Build history of the part. All positions in model axes, mm. A direction names the side the tool comes from. Round coordinates to 2 decimals unless told otherwise and drop trailing zeros. Write each loop counter-clockwise with the first axis right and the second up, starting at its lowest first coordinate (ties: lowest second). Pieces come first, ordered by that corner, then holes. Notation, with made-up numbers: (-5, 84) -> (1, 84) arc R5 cw to (1, 88) -> close; hole circle Ø9 at (-40, 25.5). An arc over 180 degrees is marked (long way). Return JSON: item names as keys, results as strings.
from build123d import *


# Not quite as in the source:
# - a fillet or chamfer that OpenCascade refuses, or shapes differently, is made with other operations: its cross-section is extruded or revolved along the edge and cut away or added


with BuildPart() as f1:
    # F0 (on Front) → F1 (revolve)
    with BuildSketch(Plane.XZ):
        Polygon((-40, 29.117645719), (-44, 29.117645719), (-44, 0), (-19, 0), (-19, -33.1176439325), (-15, -33.1176439325), (-15, 4), (-40, 4), align=None)
    revolve(axis=Axis((0, 0, -0.9199753404), (0, 0, -1)))

    # F2: fillet of radius 5 on 1 edges, made by hand

    # F2_s1 → F2_t2 (revolve, cut)
    with BuildSketch(Plane.XZ):
        with BuildLine():
            ThreePointArc((-40, 29.117645719), (-42.8729833462, 27.3809438936), (-44, 24.2186662334))
            Line((-44, 24.2186662334), (-44, 29.117645719))
            Line((-44, 29.117645719), (-40, 29.117645719))
        make_face()
    revolve(axis=Axis((0, 0, 29.117645719), (0, 0, -1)), mode=Mode.SUBTRACT)


solid = f1.part
Q1. Saw through at A-A on x = 0. List the corners of the cut face in (y, z), then the cut area to 3 significant figures.
Verdict:
{"outline": "(-44, 0) -> (-19, 0) -> (-19, -33.12) -> (-15, -33.12) -> (-15, 4) -> (-40, 4) -> (-40, 29.12) arc R5 ccw to (-44, 24.22) -> close; (15, -33.12) -> (19, -33.12) -> (19, 0) -> (44, 0) -> (44, 24.22) arc R5 ccw to (40, 29.12) -> (40, 4) -> (15, 4) -> close", "area": "688 mm²"}
Q2. Pin check, flat tips, straight feed: pin 1 Ø4 at (y, z) = (-35, -3) entering from -X; pin 2 Ø10 at (x, y) = (-8.5, -26) entering from -Z; pin 3 Ø8 at (x, y) = (1, 28) entering from +Z; pin 4 Ø1.5 at (y, z) = (7.5, -22) entering from -X. Stop position of each tip, or through.
Verdict:
{"pin 1": "passes through", "pin 2": "stops at z = 0", "pin 3": "stops at z = 4", "pin 4": "stops at x = -17.76"}
Q3. Saw through at C-C on z = 13.5. List the corners of the cut face in (x, y).
Verdict:
{"outline": "circle Ø88 at (0, 0); hole circle Ø80 at (0, 0)"}
Q4. Two-plate mould, pull along X, no slides. Class faces 3 (the cylindrical face through (-8.767, -16.856, -16.791)), 4 (the flat face through (-9, -19, 0)), 5 (the cylindrical face through (8.67, -39.05, 16.73)): +X half, -X half, draft (parallel to the pull), parting line (faces both ways), or undercut.
Verdict:
{"face 3": "parting line", "face 4": "draft", "face 5": "undercut"}
Q5. Saw through at D-D on z = -16.5. List the corners of the cut face in (x, y).
Verdict:
{"outline": "circle Ø38 at (0, 0); hole circle Ø30 at (0, 0)"}
Q6. 3-axis set-ups, long thin cutter, end or side, ignore diameter. For faces 1 (the cylindrical face through (9.538, -42.954, 11.94)), 2 (the flat face through (17, 1, 4)): which of +Z, -Z, +X, -X, +Y, -Y reach the whole face in a straight line?
Verdict:
{"face 1": "+Z, -Z", "face 2": "+Z"}
Q7. Wall check: L1, parallel to Y at x = 0, z = -8; L2, parallel to Y at x = 0, z = 19; L3, parallel to Z at x = -16, y = 9. Give the ranges that are in metal, low to high.
Verdict:
{"L1": "y = -19 to -15, 15 to 19", "L2": "y = -44 to -40, 40 to 44", "L3": "z = -33.12 to 4"}
